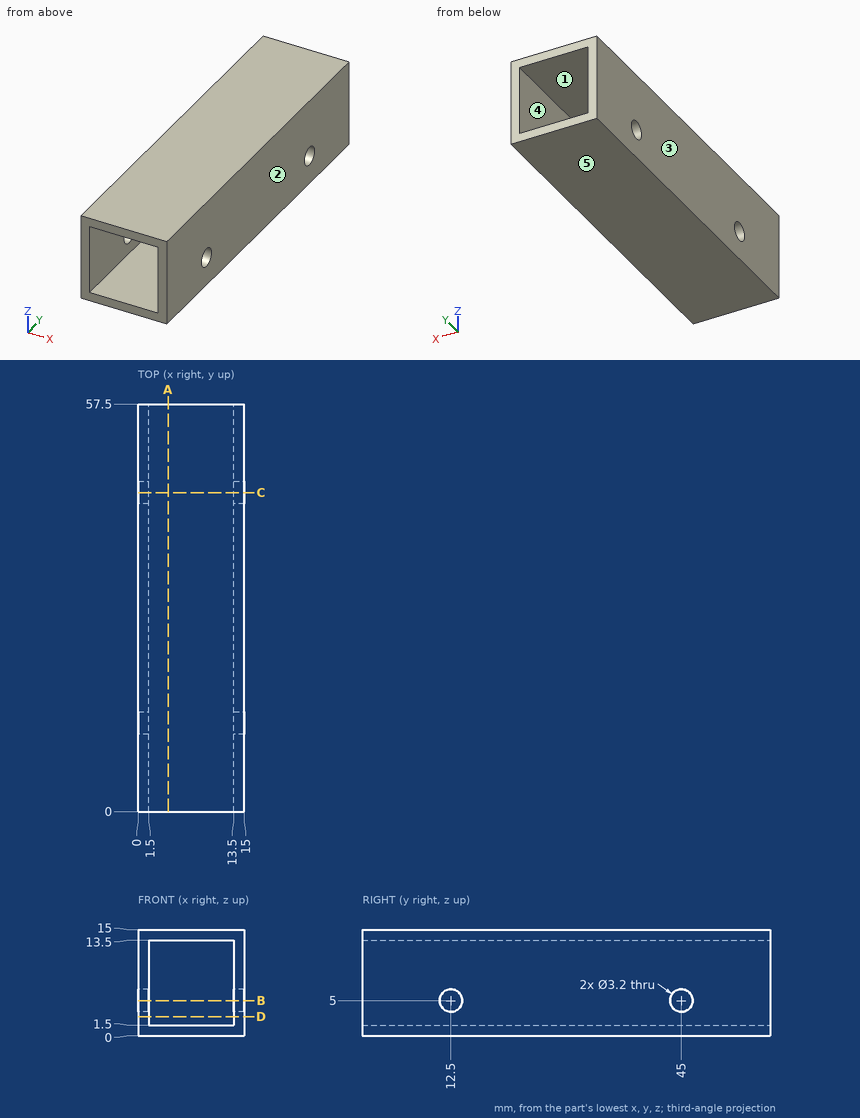
Geometry: see drawing. Coordinates: mm, zero at the bounding-box minimum. A direction names the side the tool comes from. Give positions to 0.01 mm unless a question says otherwise; leave off trailing zeros. Loops run counter-clockwise (first coordinate to the right, second up) from the corner with the lowest first, then second, coordinate; pieces in that order, holes last. Notation, with made-up numbers: (30, 80.25) - (46, 80.25) arc R19 ccw to (46, 101.25) - close; hole circle Ø6 at (77, 57.25). An arc over 180 degrees is marked (long way). Use CSV: the item, a comma, the result in double quotes. Start each with the question number.
1. Section B-B (z = 5). Output: boundary loops of the cut face in (x, y).
2. Pin query (flat end, axial travel): pin 1 (5 mm diameter, centred on x = 9, z = 8.5, fed in from -Y). Return the tip coordinate at first contact, or that it passes through.
3. Draft query along X for the marked faces 1, 2 and 3. Return one class per face: +X half, -X half, draft (parallel to the pull), parting line (faces both ways), or undercut.
4. Section A-A (x = 4.25). Output: boundary loops of the cut face in (y, z), then the cut area to 4 significant figures.
5. Reachability of the marked faces 4 and 5 from +Z, -Z, +X, -X, +Y, -Y: full face, straight path, thin tool, end or side. Return the list, or none.
6. Ray query, L1, parallel to Y at x = 1, z = 5; L2, parallel to X at y = 54, z = 4.5. Return the intervals inside material, ascending.
7. Section D-D (z = 2.75). Output: boundary loops of the cut face in (x, y).
8. Section C-C (y = 45). Output: boundary loops of the cut face in (x, z), then the cut area to 3 significant figures.
Response:
1,outline,"(0, 0) - (1.5, 0) - (1.5, 10.9) - (0, 10.9) - close; (0, 14.1) - (1.5, 14.1) - (1.5, 43.4) - (0, 43.4) - close; (0, 46.6) - (1.5, 46.6) - (1.5, 57.5) - (0, 57.5) - close; (13.5, 0) - (15, 0) - (15, 10.9) - (13.5, 10.9) - close; (13.5, 14.1) - (15, 14.1) - (15, 43.4) - (13.5, 43.4) - close; (13.5, 46.6) - (15, 46.6) - (15, 57.5) - (13.5, 57.5) - close"
2,pin 1,"through"
3,face 1,"undercut"
3,face 2,"+X half"
3,face 3,"-X half"
4,outline,"(0, 0) - (57.5, 0) - (57.5, 1.5) - (0, 1.5) - close; (0, 13.5) - (57.5, 13.5) - (57.5, 15) - (0, 15) - close"
4,area,"172.5 mm²"
5,face 4,"+Y, -Y"
5,face 5,"-Z, +X, -X, +Y, -Y"
6,L1,"0 to 10.9, 14.1 to 43.4, 46.6 to 57.5"
6,L2,"0 to 1.5, 13.5 to 15"
7,outline,"(0, 0) - (1.5, 0) - (1.5, 57.5) - (0, 57.5) - close; (13.5, 0) - (15, 0) - (15, 57.5) - (13.5, 57.5) - close"
8,outline,"(0, 0) - (15, 0) - (15, 3.4) - (13.5, 3.4) - (13.5, 1.5) - (1.5, 1.5) - (1.5, 3.4) - (0, 3.4) - close; (0, 6.6) - (1.5, 6.6) - (1.5, 13.5) - (13.5, 13.5) - (13.5, 6.6) - (15, 6.6) - (15, 15) - (0, 15) - close"
8,area,"71.4 mm²"
